For this review, take the finished solid that the model builds, in its own axes (mm). Face numbers are marked on the shaded views. A direction names the side the tool comes from. Round coordinates to 2 decimals unless told otherwise and drop trailing zeros. Loops run counter-clockwise (first coordinate to the right, second up) from the corner with the lowest first, then second, coordinate; pieces in that order, holes last. Notation, with made-up numbers: (30.5, -37) -> (82.5, -37) arc R20 ccw to (82.5, 1) -> close; hole circle Ø6 at (-30, 44.5). An arc over 180 degrees is marked (long way). Write each question's results on one line, items separated by ' | '.
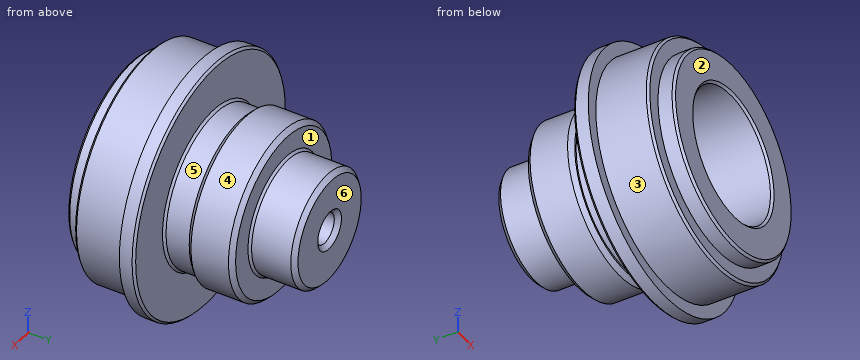
```python
from build123d import *

# Parameters (mm, degrees)
CHAMFER2_SIZE = 1
CHAMFER3_SIZE = 1
CHAMFER4_SIZE = 0.5


with BuildPart() as part:
    # Sketch1 → Revolve1 (revolve)
    with BuildSketch(Plane.XY):
        Polygon((0, 28), (0, 26.629648104), (14.528640902, 26.629648104), (14.528640902, 0), (21.838640902, 0), (21.838640902, 3.65), (25.35, 3.65), (25.35, 15.45), (28.147407407, 15.45), (28.147407407, 18.8), (17.25, 18.8), (17.25, 24.8), (18.75, 24.8), (18.75, 35.2), (12.68, 35.2), (12.68, 45.5), (3.38, 45.5), (3.38, 28), align=None)
    revolve(axis=Axis((0, 0, 0), (0, 1, 0)))

    # Chamfer2
    chamfer2_edges = [part.edges().sort_by_distance(p)[0] for p in [
        (-3.38, 45.5, 0),
        (-18.75, 35.2, 0),
        (-18.75, 24.8, 0),
    ]]
    chamfer(chamfer2_edges, length=CHAMFER2_SIZE)

    # Chamfer3
    chamfer3_edges = [part.edges().sort_by_distance(p)[0] for p in [
        (-12.68, 45.5, 0),
    ]]
    chamfer(chamfer3_edges, length=CHAMFER3_SIZE)

    # Chamfer4
    chamfer4_edges = [part.edges().sort_by_distance(p)[0] for p in [
        (-12.68, 35.2, 0),
        (-17.25, 18.8, 0),
        (-28.147407407, 18.8, 0),
        (-25.35, 3.65, 0),
        (-21.838640902, 0, 0),
        (-14.528640902, 0, 0),
    ]]
    chamfer(chamfer4_edges, length=CHAMFER4_SIZE)


solid = part.part
```
1. Consider section B-B (y = 12.5). State the section outline as (x, z) points, plus the area to 3 significant figures.
Values found:
outline: circle Ø50.7 at (0, 0); hole circle Ø29.06 at (0, 0) | area: 1,360 mm2
2. Tool access review of the marked faces 1, 2 and 3: name each direction out of +Z, -Z, +X, -X, +Y, -Y from which nothing blocks a thin tool from reaching the whole face with its end or side.
Values found:
face 1: +Y | face 2: +Z, -Z, +X, -X, -Y | face 3: -Y
3. To check wall thickness, follow probe 1 along X at (y, z) = (20.25, 0); probe 2 along X at (y, z) = (7.5, 0). State the ranges of each line that lie inside material, in increasing order.
Values found:
probe 1: x = -17.25 to -14.53, 14.53 to 17.25 | probe 2: x = -25.35 to -14.53, 14.53 to 25.35
4. Draft analysis for pull direction Y (two halves, no side actions). For the marked faces 4, 5 and 6, state which applies: released by +Y, released by -Y, zero draft, split by the parting line, or undercut.
Values found:
face 4: zero draft | face 5: undercut | face 6: released by +Y
5. For pin 1 (1 mm diameter, centred on y = 18.5, z = 18.5, fed in from +X); pin 2 (3.5 mm diameter, centred on x = -1, z = -0.5, fed in from +Y); pin 3 (8 mm diameter, centred on y = 7.5, z = -8, fed in from -X), all flat-tipped, find the tip position at first contact; note any pin that passes through.
Values found:
pin 1: stops at x = 21.6 | pin 2: stops at y = 28 | pin 3: stops at x = -25.03
6. Consider section A-A (y = 36.5). State the section outline as (x, z) points, plus the area to 3 significant figures.
Values found:
outline: circle Ø25.36 at (0, 0); hole circle Ø6.76 at (0, 0) | area: 469 mm2
